Input: dimensioned drawing with shaded views. Units: mm. Origin: part minimum x, y, z. A direction names the side the tool comes from. Round coordinates to 2 decimals unless told otherwise and drop trailing zeros. Loops run counter-clockwise (first coordinate to the right, second up) from the corner with the lowest first, then second, coordinate; pieces in that order, holes last. Notation, with made-up numbers: (-12.75, 40) - (-1.75, 40) arc R19 ccw to (-1.75, 49) - close; hole circle Ø8 at (-5, 19.5). An arc over 180 degrees is marked (long way). Write each question's results on one line, items separated by ' | '.
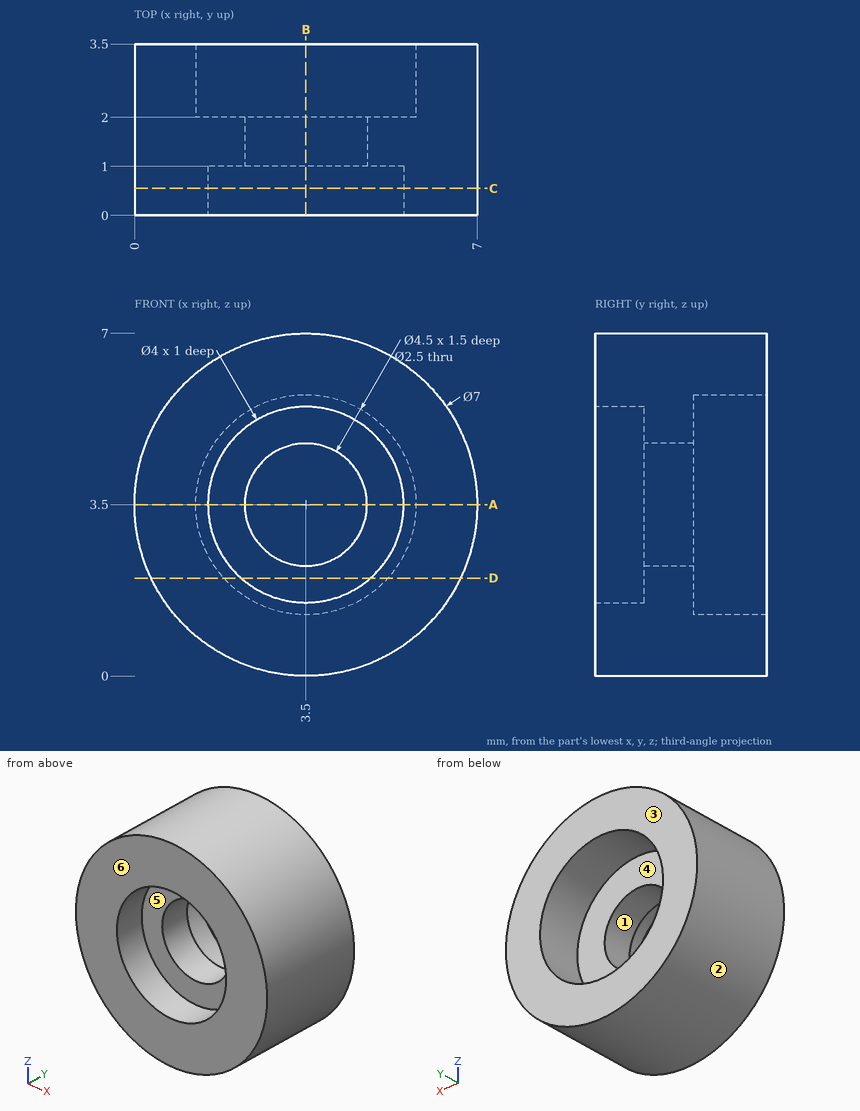
1. Contact query for flat-ended pins moving along their axis: pin 1 (2 mm diameter, centred on x = 4, z = 4, fed in from +Y); pin 2 (3 mm diameter, centred on x = 3.5, z = 3.5, fed in from -Y). Output: stop coordinate, or through.
Answer:
pin 1: y = 2 | pin 2: y = 1
2. Section query C-C, the plane y = 0.55. Output: boundary loops of the cut face in (x, z), plus the area to 3 significant figures.
Answer:
outline: circle Ø7 at (3.5, 3.5); hole circle Ø4 at (3.5, 3.5) | area: 25.9 mm^2
3. Section query D-D, the plane z = 2. Output: boundary loops of the cut face in (x, y), plus the area to 3 significant figures.
Answer:
outline: (0.34, 0) - (2.18, 0) - (2.18, 1) - (4.82, 1) - (4.82, 0) - (6.66, 0) - (6.66, 3.5) - (5.18, 3.5) - (5.18, 2) - (1.82, 2) - (1.82, 3.5) - (0.34, 3.5) - close | area: 14.5 mm^2
4. Section query A-A, the plane z = 3.5. Output: boundary loops of the cut face in (x, y).
Answer:
outline: (0, 0) - (1.5, 0) - (1.5, 1) - (2.25, 1) - (2.25, 2) - (1.25, 2) - (1.25, 3.5) - (0, 3.5) - close; (4.75, 1) - (5.5, 1) - (5.5, 0) - (7, 0) - (7, 3.5) - (5.75, 3.5) - (5.75, 2) - (4.75, 2) - close
5. Line query: line 1 (X direction, y = 1.2, z = 3.5); line 2 (X direction, y = 0.6, z = 3.5); line 3 (Z direction, x = 4.5, y = 0.8). Output: solid intervals per line, ascending. Write a range as [from, to].
Answer:
line 1: [0, 2.25], [4.75, 7] | line 2: [0, 1.5], [5.5, 7] | line 3: [0.15, 1.77], [5.23, 6.85]
6. Set-up query: the marked faces 4, 5 and 6. Return all of +Z, -Z, +X, -X, +Y, -Y with unobstructed straight access to the full face (end or side cutting, diameter ignored); none if empty.
Answer:
face 4: +Y | face 5: -Y | face 6: +Z, -Z, +X, -X, -Y
7. Mould query, pull axis Z, two halves, no side actions, for the marked faces 1, 2 and 3. Classes: pulls with the +Z half, pulls with the -Z half, needs draft (parallel to the pull), parting line crosses it, or undercut.
Answer:
face 1: undercut | face 2: parting line crosses it | face 3: needs draft
8. Section query B-B, the plane x = 3.5. Output: boundary loops of the cut face in (y, z).
Answer:
outline: (0, 0) - (3.5, 0) - (3.5, 1.25) - (2, 1.25) - (2, 2.25) - (1, 2.25) - (1, 1.5) - (0, 1.5) - close; (0, 5.5) - (1, 5.5) - (1, 4.75) - (2, 4.75) - (2, 5.75) - (3.5, 5.75) - (3.5, 7) - (0, 7) - close
